Work out the finished part from the listing and answer in its coordinate system (mm). A direction names the side the tool comes from. Give positions to 0.01 mm unless a question says otherwise; leave off trailing zeros. Loops run counter-clockwise (first coordinate to the right, second up) from the corner with the lowest first, then second, coordinate; pieces in that order, holes last. Notation, with made-up numbers: (-24, -26.5) -> (23, -26.5) arc R4 ccw to (23, -22.5) -> close; hole circle Ø10 at (54.25, -21.5). An arc over 180 degrees is marked (long way). Answer as CSV lines item,"result". Start each with the question number.
1. Find the intervals of material crossed by line 1 along Z through (x, y) = (6.25, 4.75); line 2 along Z through (x, y) = (5.5, -1); line 3 along Y through (x, z) = (3.5, 4.5), in increasing order.
2. Find section C-C, the plane z = 5.75. Give the vertices of the cut face in (x, y).
3. Find section A-A, the plane x = 0. Give the vertices of the cut face in (y, z), and give its area (3 significant figures).
4. Flat-ended cylindrical pins translate along their axes: pin 1 Ø3 at (x, z) = (5, 1) entering from -Y; pin 2 Ø1 at (y, z) = (5, 1.5) entering from -X. Find the tip coordinate at first contact, or state that the pin passes through.
5. A tool of negligible diameter and unlimited length cuts with its end or side. For faces 1 (the face through (-0.75, 5.7, 2.49)), 2 (the face through (0, 0, 6.5)), from which of +Z, -Z, +X, -X, +Y, -Y can it reach the whole face along a straight path? Write none if from no direction.
6. Find section D-D, the plane z = 2.75. Give the vertices of the cut face in (x, y), and give its area (3 significant figures).
from build123d import *

# Parameters (mm, degrees)
F0_R     = 9
F1_DEPTH = 2
F2_R     = 5.75
F3_DEPTH = 1
F4_R     = 4.15
F5_DEPTH = 3.5
F6_R     = 0.75
F7_SIZE2 = 2
F7_SIZE  = 0.4


with BuildPart() as f1:
    # F0 (on Top) → F1 (new body)
    with BuildSketch(Plane.XY):
        Circle(F0_R)
    extrude(amount=F1_DEPTH)

    # F2 (on face) → F3 (join)
    with BuildSketch(Plane.XY.offset(2)):
        Circle(F2_R)
    extrude(amount=F3_DEPTH)

    # F4 (on face) → F5 (join)
    with BuildSketch(Plane.XY.offset(3)):
        Circle(F4_R)
    extrude(amount=F5_DEPTH)

    # F6
    f6_edges = [f1.edges().sort_by_distance(p)[0] for p in [
        (-9, 0, 0),
    ]]
    fillet(f6_edges, radius=F6_R)

    # F7
    f7_edges = [f1.edges().sort_by_distance(p)[0] for p in [
        (-4.15, 0, 6.5),
    ]]
    f7_side = f1.faces().sort_by_distance((0, 0, 6.5))[0]
    chamfer(f7_edges, length=F7_SIZE, length2=F7_SIZE2, reference=f7_side)


solid = f1.part
Resolved:
1,line 1,"z = 0 to 2"
1,line 2,"z = 0 to 3"
1,line 3,"y = -2.23 to 2.23"
2,outline,"circle Ø7.8 at (0, 0)"
3,outline,"(-9, 0.75) arc R0.75 ccw to (-8.25, 0) -> (8.25, 0) arc R0.75 ccw to (9, 0.75) -> (9, 2) -> (5.75, 2) -> (5.75, 3) -> (4.15, 3) -> (4.15, 4.5) -> (3.75, 6.5) -> (-3.75, 6.5) -> (-4.15, 4.5) -> (-4.15, 3) -> (-5.75, 3) -> (-5.75, 2) -> (-9, 2) -> close"
3,area,"75.5 mm^2"
4,pin 1,"stops at y = -8.29"
4,pin 2,"stops at x = -7.79"
5,face 1,"+Z"
5,face 2,"+Z, +X, -X, +Y, -Y"
6,outline,"circle Ø11.5 at (0, 0)"
6,area,"104 mm^2"
